```python
from build123d import *

# Parameters (mm, degrees)
CROQUIS1_R              = 3.1
SALIENTE_EXTRUIR1_DEPTH = 3.935
SALIENTE_EXTRUIR2_START = 0.85
CROQUIS1_3_R            = 3.1
CROQUIS1_3_R_2          = 2.5
SALIENTE_EXTRUIR2_DEPTH = 2.235


with BuildPart() as part:
    # Croquis1 → Saliente-Extruir1 (new body)
    with BuildSketch(Plane(origin=(0, 0, 0), x_dir=(1, 0, 0), z_dir=(0, 1, 0))):
        with BuildLine():
            Line((0, 4), (84.76, 4))
            ThreePointArc((84.76, 4), (88.76, 0), (84.76, -4))
            Line((84.76, -4), (0, -4))
            ThreePointArc((0, -4), (-4, 0), (0, 4))
        make_face()
        with Locations(Location((0, 0, 0), (0, 0, 270))):
            Circle(CROQUIS1_R, mode=Mode.SUBTRACT)
        with Locations(Location((84.76, 0, 0), (0, 0, 270))):
            Circle(CROQUIS1_R, mode=Mode.SUBTRACT)
        with Locations(Location((42.38, 0, 0), (0, 0, 270))):
            Circle(CROQUIS1_R, mode=Mode.SUBTRACT)
    extrude(amount=SALIENTE_EXTRUIR1_DEPTH)

    # Croquis1<3> → Saliente-Extruir2 (add)
    # profile 1 of 3: a face of its own
    with BuildSketch(Plane(origin=(0, 0, 0), x_dir=(1, 0, 0), z_dir=(0, 1, 0)).offset(SALIENTE_EXTRUIR2_START)):
        with Locations(Location((0, 0, 0), (0, 0, 270))):
            Circle(CROQUIS1_3_R)
        with Locations(Location((0, 0, 0), (0, 0, 270))):
            Circle(CROQUIS1_3_R_2, mode=Mode.SUBTRACT)
    # profile 2 of 3: a face of its own
    with BuildSketch(Plane(origin=(0, 0, 0), x_dir=(1, 0, 0), z_dir=(0, 1, 0)).offset(SALIENTE_EXTRUIR2_START)):
        with Locations(Location((84.76, 0, 0), (0, 0, 270))):
            Circle(CROQUIS1_3_R)
        with Locations(Location((84.76, 0, 0), (0, 0, 270))):
            Circle(CROQUIS1_3_R_2, mode=Mode.SUBTRACT)
    # profile 3 of 3: a face of its own
    with BuildSketch(Plane(origin=(0, 0, 0), x_dir=(1, 0, 0), z_dir=(0, 1, 0)).offset(SALIENTE_EXTRUIR2_START)):
        with Locations(Location((42.38, 0, 0), (0, 0, 270))):
            Circle(CROQUIS1_3_R)
        with Locations(Location((42.38, 0, 0), (0, 0, 270))):
            Circle(CROQUIS1_3_R_2, mode=Mode.SUBTRACT)
    extrude(amount=SALIENTE_EXTRUIR2_DEPTH)


solid = part.part
```
Source: CAD feature listing. Evaluate the final solid. Frame: model axes, mm. A direction names the side the tool comes from. Give positions to 0.01 mm unless a question says otherwise; leave off trailing zeros. Put each result on its own line as item: value. Start each with the question number.
1) Contact query for flat-ended pins moving along their axis: P1, Ø1.9, axis at x = 83, z = 0.5, coming from the -Y side; P2, Ø3, axis at x = 83.5, z = -0.5, coming from the +Y side (3 decimals). Output: stop coordinate, or through.
2) Cut plane A-A (z = 0). State how many separate pieces and enclosed holes the cut face has, then the cut area to 3 significant figures.
3) Material intervals for probe 1 along X at (y, z) = (0.6, 0); probe 2 along X at (y, z) = (1.3, 0.25); probe 3 along Z at (x, y) = (45, 0.25), sorted ascending.
4) Reachability of faces 1 (the face through (0.931, 3.504, 2.957)), 2 (the face through (-4, 2, 0)), 3 (the face through (39.354, 0.419, -0.672)) from +Z, -Z, +X, -X, +Y, -Y: full face, straight path, thin tool, end or side. Return the list, or none.
Results are:
1. P1: stops at y = 0.85
1. P2: stops at y = 3.085
2. separate pieces: 4
2. enclosed holes: 0
2. area: 300 mm2
3. probe 1: x = -4 to -3.1, 3.1 to 39.28, 45.48 to 81.66, 87.86 to 88.76
3. probe 2: x = -3.99 to -2.49, 2.49 to 39.89, 44.87 to 82.27, 87.25 to 88.75
3. probe 3: z = -4 to -1.66, 1.66 to 4
4. face 1: +Y
4. face 2: -X, +Y, -Y
4. face 3: -Y
